Here's how the part is built. I have some questions about the finished solid (model axes, mm). A direction names the side the tool comes from. Round coordinates to 2 decimals unless told otherwise and drop trailing zeros. Order: outer loops, then holes, each group sorted by start corner. A loop starts at its lowest first (then second) coordinate and runs counter-clockwise, first axis right, second up. Notation, with made-up numbers: (89, 49) -> (139, 49) arc R7 cw to (139, 62) -> close; hole circle Ø9 at (-32, 81.5). An arc over 180 degrees is marked (long way). Use a Markdown table: item, result. Add a question column.
(1) I want a section at C-C, the plane x = 20. Please give me the cut outline in (y, z), then the cut area to 3 significant figures.
(2) I want a section at D-D, the plane z = 15. Please give me the cut outline in (x, y), then the cut area to 3 significant figures.
(3) If I drill on probe 1 along Z at (x, y) = (1, 20.5); probe 2 along Z at (x, y) = (-0.5, 8); probe 3 along X at (y, z) = (29, -14.5), over which ranges is the centre line in solid material (lowest first)?
(4) Thinking about a two-plate mould opening in Y: for faces 1 (the face through (-4.5, 6, -52)), 2 (the face through (-5, 16, -20.45)), 3 (the face through (-24, 45, 27)), which applies, pulls with the +Y half, pulls with the -Y half, needs draft (parallel to the pull), parting line crosses it, or undercut?
(5) I want a section at A-A, the plane x = 0. Give the number of separate pieces and of enclosed holes in the cut face, then the cut area to 3 significant figures.
(6) On a 3-axis mill with a long thin cutter (end or side, diameter ignored), from which of +Z, -Z, +X, -X, +Y, -Y can I reach the whole of each face in a straight line? I mean faces 4 (the face through (-22, 45, 24)), 5 (the face through (-10.25, 16, 0)), 6 (the face through (0, 11, -52)), 7 (the face through (10, 16, -23.45)). Say none if no direction works.
(7) I'm going to push flat-ended pins straight in: P1, Ø3.5, axis at x = -5, z = 24.5, coming from the +Y side; P2, Ø22.5, axis at y = 20, z = -0.5, coming from the -X side; P3, Ø1.5, axis at x = 1.5, y = 17.5, coming from the +Z side. Where does each tip first touch, or does it pass through?
(8) I want a section at B-B, the plane y = 31.5. Please give me the cut outline in (x, z).
from build123d import *

# Parameters (mm, degrees)
CROQUIS2_R              = 1.45
SALIENTE_EXTRUIR1_DEPTH = 2
CROQUIS3_W              = 26.5
CROQUIS3_H              = 46.9
CROQUIS3_W_2            = 20.5
CROQUIS3_H_2            = 40.9
SALIENTE_EXTRUIR2_DEPTH = 28.1
SALIENTE_EXTRUIR3_DEPTH = 3.5
CROQUIS5_R              = 1.45
CORTAR_EXTRUIR1_DEPTH   = 48.534565862
CROQUIS6_W              = 9
CROQUIS6_H              = 24
CORTAR_EXTRUIR2_DEPTH   = 3.5
CROQUIS7_R              = 45
SALIENTE_EXTRUIR4_DEPTH = 2
CROQUIS8_R              = 45
CROQUIS8_R_2            = 40
SALIENTE_EXTRUIR5_DEPTH = 43
CROQUIS9_R              = 43.5
CROQUIS9_R_2            = 41.5
CORTAR_EXTRUIR3_DEPTH   = 30
CROQUIS10_W             = 9
CROQUIS10_H             = 9
CORTAR_EXTRUIR4_DEPTH   = 87.409541035
CROQUIS11_R             = 1.45
CORTAR_EXTRUIR5_DEPTH   = 84.05905068


with BuildPart() as part:
    # Croquis2 → Saliente-Extruir1 (new body)
    with BuildSketch(Plane(origin=(0, 0, 0), x_dir=(1, 0, 0), z_dir=(0, 1, 0))):
        with BuildLine():
            Line((-23.45, 5), (-23.45, -5))
            ThreePointArc((-23.45, -5), (-22.439518395, -7.439518395), (-20, -8.45))
            Line((-20, -8.45), (-13.25, -8.45))
            Line((-13.25, -8.45), (-13.25, -23.45))
            Line((-13.25, -23.45), (13.25, -23.45))
            Line((13.25, -23.45), (13.25, -8.45))
            Line((13.25, -8.45), (20, -8.45))
            ThreePointArc((20, -8.45), (22.439518395, -7.439518395), (23.45, -5))
            Line((23.45, -5), (23.45, 5))
            ThreePointArc((23.45, 5), (22.439518395, 7.439518395), (20, 8.45))
            Line((20, 8.45), (13.25, 8.45))
            Line((13.25, 8.45), (13.25, 23.45))
            Line((13.25, 23.45), (-13.25, 23.45))
            Line((-13.25, 23.45), (-13.25, 8.45))
            Line((-13.25, 8.45), (-20, 8.45))
            ThreePointArc((-20, 8.45), (-22.439518395, 7.439518395), (-23.45, 5))
        make_face()
        with Locations(Location((-20, 5, 0), (0, 0, 270))):
            Circle(CROQUIS2_R, mode=Mode.SUBTRACT)
        with Locations(Location((-20, -5, 0), (0, 0, 90))):
            Circle(CROQUIS2_R, mode=Mode.SUBTRACT)
        with Locations(Location((20, -5, 0), (0, 0, 270))):
            Circle(CROQUIS2_R, mode=Mode.SUBTRACT)
        with Locations(Location((20, 5, 0), (0, 0, 90))):
            Circle(CROQUIS2_R, mode=Mode.SUBTRACT)
        with Locations(Location((-20, 0, 0), (0, 0, 270))):
            Circle(CROQUIS2_R, mode=Mode.SUBTRACT)
        with Locations(Location((20, 0, 0), (0, 0, 90))):
            Circle(CROQUIS2_R, mode=Mode.SUBTRACT)
    extrude(amount=SALIENTE_EXTRUIR1_DEPTH)

    # Croquis3 → Saliente-Extruir2 (add)
    with BuildSketch(Plane(origin=(0, 2, 0), x_dir=(1, 0, 0), z_dir=(0, 1, 0))):
        Rectangle(CROQUIS3_W, CROQUIS3_H)
        Rectangle(CROQUIS3_W_2, CROQUIS3_H_2, mode=Mode.SUBTRACT)
    extrude(amount=SALIENTE_EXTRUIR2_DEPTH)

    # Croquis4 → Saliente-Extruir3 (add)
    with BuildSketch(Plane(origin=(0, 30.1, 0), x_dir=(1, 0, 0), z_dir=(0, 1, 0))):
        with BuildLine():
            Line((-5, 28.348235425), (5, 28.348235425))
            ThreePointArc((5, 28.348235425), (8.069980707, 26.820373751), (8.702217698, 23.45))
            Line((8.702217698, 23.45), (-8.702217698, 23.45))
            ThreePointArc((-8.702217698, 23.45), (-8.069980707, 26.820373751), (-5, 28.348235425))
        make_face()
        with BuildLine():
            Line((-8.702217698, -23.45), (8.702217698, -23.45))
            ThreePointArc((8.702217698, -23.45), (8.069980707, -26.820373751), (5, -28.348235425))
            Line((5, -28.348235425), (-5, -28.348235425))
            ThreePointArc((-5, -28.348235425), (-8.069980707, -26.820373751), (-8.702217698, -23.45))
        make_face()
    extrude(amount=-SALIENTE_EXTRUIR3_DEPTH)

    # Croquis5 → Cortar-Extruir1 (cut, through all)
    with BuildSketch(Plane(origin=(0, 30.1, 0), x_dir=(1, 0, 0), z_dir=(0, 1, 0))):
        with Locations(Location((-5, 24.5, 0), (0, 0, 270))):
            Circle(CROQUIS5_R)
        with Locations(Location((5, 24.5, 0), (0, 0, 313.602818973))):
            Circle(CROQUIS5_R)
        with Locations(Location((5, -24.5, 0), (0, 0, 270))):
            Circle(CROQUIS5_R)
        with Locations(Location((-5, -24.5, 0), (0, 0, 133.602818973))):
            Circle(CROQUIS5_R)
    extrude(amount=-CORTAR_EXTRUIR1_DEPTH, mode=Mode.SUBTRACT)

    # Croquis6 → Cortar-Extruir2 (cut)
    with BuildSketch(Plane(origin=(0, 0, -23.45), x_dir=(-1, 0, 0), z_dir=(0, 0, -1))):
        with Locations((0, 14)):
            Rectangle(CROQUIS6_W, CROQUIS6_H)
    extrude(amount=-CORTAR_EXTRUIR2_DEPTH, mode=Mode.SUBTRACT)

    # Croquis7 → Saliente-Extruir4 (add)
    with BuildSketch(Plane.XZ):
        with Locations(Location((0, -9.998235425, 0), (0, 0, 270))):
            Circle(CROQUIS7_R)
    extrude(amount=-SALIENTE_EXTRUIR4_DEPTH)

    # Croquis8 → Saliente-Extruir5 (add)
    with BuildSketch(Plane(origin=(0, 2, 0), x_dir=(1, 0, 0), z_dir=(0, 1, 0))):
        with Locations(Location((0, 9.998235425, 0), (0, 0, 90))):
            Circle(CROQUIS8_R)
        with Locations(Location((0, 9.998235425, 0), (0, 0, 270))):
            Circle(CROQUIS8_R_2, mode=Mode.SUBTRACT)
    extrude(amount=SALIENTE_EXTRUIR5_DEPTH)

    # Croquis9 → Cortar-Extruir3 (cut)
    with BuildSketch(Plane(origin=(0, 45, 0), x_dir=(1, 0, 0), z_dir=(0, 1, 0))):
        with Locations(Location((0, 9.998235425, 0), (0, 0, 270))):
            Circle(CROQUIS9_R)
        with Locations(Location((0, 9.998235425, 0), (0, 0, 270))):
            Circle(CROQUIS9_R_2, mode=Mode.SUBTRACT)
    extrude(amount=-CORTAR_EXTRUIR3_DEPTH, mode=Mode.SUBTRACT)

    # Croquis10 → Cortar-Extruir4 (cut, through all)
    with BuildSketch(Plane(origin=(0, 0, -23.45), x_dir=(-1, 0, 0), z_dir=(0, 0, -1))):
        with Locations((0, 6.5)):
            Rectangle(CROQUIS10_W, CROQUIS10_H)
    extrude(amount=CORTAR_EXTRUIR4_DEPTH, mode=Mode.SUBTRACT)

    # Croquis11 → Cortar-Extruir5 (cut, through all)
    with BuildSketch(Plane(origin=(0, 2, 0), x_dir=(1, 0, 0), z_dir=(0, 1, 0))):
        with Locations(Location((-20, 9.998235425, 0), (0, 0, 270))):
            Circle(CROQUIS11_R)
        with Locations(Location((20, 9.998235425, 0), (0, 0, 90))):
            Circle(CROQUIS11_R)
    extrude(amount=-CORTAR_EXTRUIR5_DEPTH, mode=Mode.SUBTRACT)


solid = part.part
Taken from the geometry:
| question | item | result |
|---|---|---|
| 1 | outline | (0, -50.31) -> (45, -50.31) -> (45, -48.63) -> (15, -48.63) -> (15, -46.36) -> (45, -46.36) -> (45, -44.64) -> (2, -44.64) -> (2, -11.45) -> (0, -11.45) -> close; (0, -8.55) -> (2, -8.55) -> (2, 24.64) -> (45, 24.64) -> (45, 26.36) -> (15, 26.36) -> (15, 28.63) -> (45, 28.63) -> (45, 30.31) -> (0, 30.31) -> close |
| 1 | area | 507 mm2 |
| 2 | outline | (-37.42, 0) -> (37.42, 0) -> (37.42, 45) -> (35.6, 45) -> (35.6, 15) -> (33.13, 15) -> (33.13, 45) -> (31.23, 45) -> (31.23, 2) -> (13.25, 2) -> (13.25, 30.1) -> (10.25, 30.1) -> (10.25, 2) -> (-10.25, 2) -> (-10.25, 30.1) -> (-13.25, 30.1) -> (-13.25, 2) -> (-31.23, 2) -> (-31.23, 45) -> (-33.13, 45) -> (-33.13, 15) -> (-35.6, 15) -> (-35.6, 45) -> (-37.42, 45) -> close |
| 2 | area | 702 mm2 |
| 3 | probe 1 | z = -54.99 to -53.49, -51.49 to -49.99, 20.45 to 23.45, 29.99 to 31.49, 33.49 to 34.99 |
| 3 | probe 2 | z = 20.45 to 23.45, 30 to 35 |
| 3 | probe 3 | x = -44.77 to -43.27, -41.26 to -39.75, -13.25 to -10.25, 10.25 to 13.25, 39.75 to 41.26, 43.27 to 44.77 |
| 4 | face 1 | undercut |
| 4 | face 2 | needs draft |
| 4 | face 3 | pulls with the +Y half |
| 5 | separate pieces | 3 |
| 5 | enclosed holes | 0 |
| 5 | area | 576 mm2 |
| 6 | face 4 | +Z, -Z, +X, -X, +Y |
| 6 | face 5 | +Y |
| 6 | face 6 | -Z |
| 6 | face 7 | none |
| 7 | P1 | stops at y = 30.1 |
| 7 | P2 | stops at x = -45 |
| 7 | P3 | stops at z = 35 |
| 8 | outline | circle Ø90 at (0, -10); circle Ø83 at (0, -10); hole circle Ø87 at (0, -10); hole circle Ø80 at (0, -10) |
